Could you check a few things on this model? Use its own coordinates, in mm. Face numbers are marked on the shaded views. A direction names the side the tool comes from. Round coordinates to 2 decimals unless told otherwise and drop trailing zeros. Order: outer loops, then holes, each group sorted by start corner. A loop starts at its lowest first (then second) coordinate and runs counter-clockwise, first axis right, second up. Notation, with made-up numbers: (28, 29) - (81, 29) arc R19 ccw to (81, 63) - close; hole circle Ø2 at (28.25, 44). An arc over 180 degrees is marked (long way). Use one line per item in the form item = value.
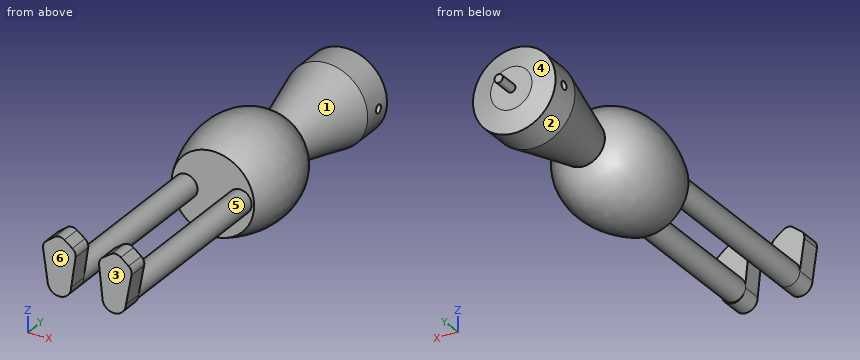
from build123d import *

# Parameters (mm, degrees)
SKETCH2_R               = 2.83366024
BOSS_EXTRUDE1_DEPTH     = 45
BOSS_EXTRUDE2_DEPTH     = 5
FILLET1_R               = 2
FILLET2_R               = 2
CUT_EXTRUDE2_DEPTH      = 115
CUT_EXTRUDE2_DEPTH_BACK = 96
SKETCH5_R               = 1
SKETCH7_R               = 1
BOSS_EXTRUDE3_DEPTH     = 5


with BuildPart() as part:
    # Sketch1 → Revolve7 (revolve)
    with BuildSketch(Plane.XY, mode=Mode.PRIVATE) as revolve7_sk:
        Polygon((0, 0), (0, 28.475188422), (-4.956233819, 28.475188422), (-9.912467638, 27.282021021), (-9.912467638, 19.643055135), (-5.183583994, 0), align=None)
        with BuildLine():
            Line((0, -25.281339493), (0, 0))
            Line((0, 0), (-5.183583994, 0))
            add(Edge.make_bspline(
                [(-5.183583994, 0), (-8.573978987, -1.188883935), (-14.492218072, -9.39255897), (-12.177190855, -19.84099189), (-9.91246763, -25.281339493)],
                knots=[0, 0, 0, 0, 0.353823056, 1, 1, 1, 1], degree=3))
            Line((-9.91246763, -25.281339493), (-4.956233811, -25.281339493))
            Line((-4.956233811, -25.281339493), (0, -25.281339493))
        make_face()
    revolve(revolve7_sk.sketch.rotate(Axis((0, 53.654641341, 0), (0, -1, 0)), 270), axis=Axis((0, 53.654641341, 0), (0, -1, 0)))

    # Sketch2 → Boss-Extrude1 (add)
    with BuildSketch(Plane.XZ.offset(25.281339493)):
        with Locations(Location((-6.497142555, 0, 0), (0, 0, 90))):
            Circle(SKETCH2_R)
        with Locations(Location((6.497142555, 0, 0), (0, 0, 90))):
            Circle(SKETCH2_R)
    extrude(amount=BOSS_EXTRUDE1_DEPTH)

    # Sketch3 → Boss-Extrude2 (add)
    with BuildSketch(Plane.XZ.offset(70.281339493)):
        with BuildLine():
            Line((-9.330802795, 0), (-10.560252354, 8.471200618))
            Line((-10.560252354, 8.471200618), (-6.497142555, 11.576029804))
            Line((-6.497142555, 11.576029804), (-2.434032757, 8.471200618))
            Line((-2.434032757, 8.471200618), (-3.663482316, 0))
            ThreePointArc((-3.663482316, 0), (-6.497142555, -2.83366024), (-9.330802795, 0))
        make_face()
        with BuildLine():
            Line((2.917036225, 8.367030218), (7.097906526, 11.311372086))
            Line((7.097906526, 11.311372086), (11.03709893, 8.050760378))
            Line((11.03709893, 8.050760378), (9.478884483, -0.366172191))
            ThreePointArc((9.478884483, -0.366172191), (6.537086047, -3.087400346), (3.815857893, -0.14560191))
            Line((3.815857893, -0.14560191), (2.917036225, 8.367030218))
        make_face()
    extrude(amount=BOSS_EXTRUDE2_DEPTH)

    # Fillet1
    fillet1_edges = [part.edges().sort_by_distance(p)[0] for p in [
        (-6.497142555, -72.781339493, 11.576029804),
        (7.097906526, -72.781339493, 11.311372086),
    ]]
    fillet(fillet1_edges, radius=FILLET1_R)

    # Fillet2
    fillet2_edges = [part.edges().sort_by_distance(p)[0] for p in [
        (-2.434032757, -72.781339493, 8.471200618),
        (-10.560252354, -72.781339493, 8.471200618),
        (11.03709893, -72.781339493, 8.050760378),
        (2.917036225, -72.781339493, 8.367030218),
    ]]
    fillet(fillet2_edges, radius=FILLET2_R)

    # Sketch5 → Cut-Extrude2 (cut, two sides: drawn at the far end of the back side and taken through both)
    with BuildSketch(Plane(origin=(0, 0, 0), x_dir=(0, 0, -1), z_dir=(1, 0, 0)).offset(-CUT_EXTRUDE2_DEPTH_BACK)):
        with Locations(Location((0, 23.936282306, 0), (0, 0, 180))):
            Circle(SKETCH5_R)
    extrude(amount=CUT_EXTRUDE2_DEPTH + CUT_EXTRUDE2_DEPTH_BACK, mode=Mode.SUBTRACT)

    # Sketch7 → Boss-Extrude3 (add)
    with BuildSketch(Plane(origin=(0, 28.475188422, 0), x_dir=(1, 0, 0), z_dir=(0, 1, 0))):
        with Locations(Location((0, 0, 0), (0, 0, 270))):
            Circle(SKETCH7_R)
    extrude(amount=BOSS_EXTRUDE3_DEPTH)


solid = part.part
Item 1: Will these pins go through, and if not, where does the flat tip stop? P1, Ø4, axis at x = 4.5, y = -55.5, coming from the -Z side; P2, Ø1.5, axis at y = -43.5, z = -2, coming from the -X side; P3, Ø5, axis at y = -31, z = -1, coming from the -X side.
Found:
P1 = -2.83
P2 = -9.04
P3 = -9.33
Item 2: For the marked faces 1, 2 and 3, which set-ups out of +Z, -Z, +X, -X, +Y, -Y let a thin tool reach every point of the face, with its end or its side?
Found:
face_1 = none
face_2 = +Y
face_3 = +Z, -Z, +X, -X, -Y
Item 3: Imagine slicing it at A-A on y = -63. Please give me the cut outline in (x, z), plus the area to 3 significant figures.
Found:
outline = circle Ø5.67 at (-6.5, 0); circle Ø5.67 at (6.5, 0)
area = 50.5 mm2
Item 4: I need wall thicknesses on L1, parallel to Y at x = -3, z = 0; L2, parallel to Y at x = 5, z = 0; L3, parallel to Z at x = 6.25, y = -44. Which ranges of each line are inside material? Lowest first, please.
Found:
L1 = -25.28 to 22.94, 24.94 to 28.48
L2 = -75.28 to 22.94, 24.94 to 28.46
L3 = -2.82 to 2.82
Item 5: If we mould it in two halves opening along Y, with no side actions, what happens to the marked faces 4, 5 and 6? For each: released by +Y, released by -Y, zero draft, split by the parting line, or undercut.
Found:
face_4 = released by +Y
face_5 = undercut
face_6 = released by -Y
